Geometry check sheet. Reference: drawing and pictorial views, mm from the part's lowest x, y, z. Give positions to 0.01 mm unless a question says otherwise; leave off trailing zeros. Write each loop counter-clockwise with the first axis right and the second up, starting at its lowest first coordinate (ties: lowest second). Pieces come first, ordered by that corner, then holes. Notation, with made-up numbers: M -7.75,-12.75 L 29.25,-12.75 A13 ccw 29.25,-2.75 Z; hole C -38.5,74 d3. An arc over 180 degrees is marked long. One line per item, written item: value. Start each with the question number.
1. Cross-section at B-B on y = 1.75. Record the cut outline in (x, z), then the cut area to 3 significant figures.
2. Cross-section at D-D on x = 58. Record the cut outline in (y, z), then the cut area to 3 significant figures.
3. Cross-section at A-A on z = 11. Record the cut outline in (x, y), then the cut area to 3 significant figures.
4. Gauge pin test, flat end, axial feed: pin 1 (0.6 mm diameter, centred on x = 9.5, y = 4, fed in from +Z). Record the tip position at first contact, or that the pin passes through.
5. Scan lines: line 1 (X direction, y = 3, z = 16); line 2 (Z direction, x = 57, y = 3.5); line 3 (Y direction, x = 58, z = 37.75). Record each from-to range of solid material in increasing order.
6. Release check for a two-part mould opening along X. For the marked faces 1, 2 and 3 record: pulls with the +X half, pulls with the -X half, needs draft (parallel to the pull), parting line crosses it, or undercut.
7. Cross-section at C-C on z = 16.5. Record the cut outline in (x, y).
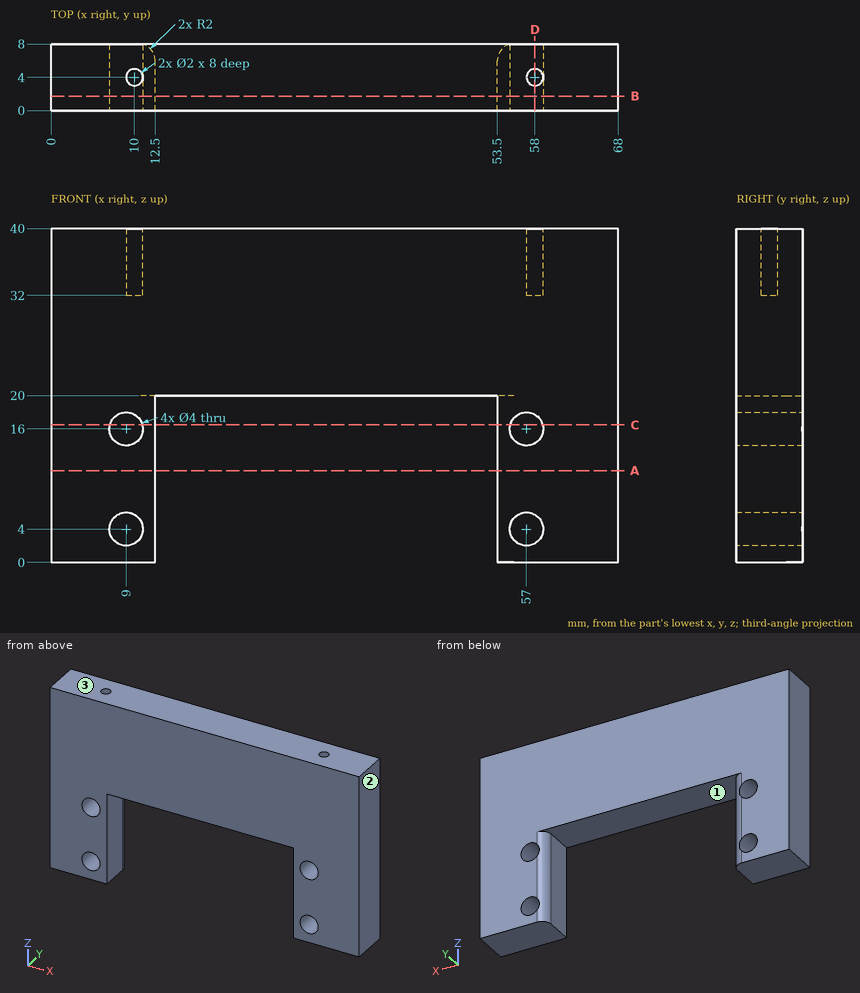
Report:
1. outline: M 0,0 L 12.5,0 L 12.5,20 L 53.5,20 L 53.5,0 L 68,0 L 68,40 L 0,40 Z; hole C 9,4 d4; hole C 9,16 d4; hole C 57,4 d4; hole C 57,16 d4
1. area: 1,850 mm^2
2. outline: M 0,0 L 8,0 L 8,2.27 L 0,2.27 Z; M 0,5.73 L 8,5.73 L 8,14.27 L 0,14.27 Z; M 0,17.73 L 8,17.73 L 8,40 L 5,40 L 5,32 L 3,32 L 3,40 L 0,40 Z
2. area: 249 mm^2
3. outline: M 0,0 L 12.5,0 L 12.5,6 A2 ccw 10.5,8 L 0,8 Z; M 53.5,0 L 68,0 L 68,8 L 55.5,8 A2 ccw 53.5,6 Z
3. area: 214 mm^2
4. pin 1: stops at z = 32
5. line 1: x = 0 to 7, 11 to 12.5, 53.5 to 55, 59 to 68
5. line 2: z = 0 to 2, 6 to 14, 18 to 40
5. line 3: y = 0 to 3, 5 to 8
6. face 1: undercut
6. face 2: pulls with the +X half
6. face 3: needs draft
7. outline: M 0,0 L 7.06,0 L 7.06,8 L 0,8 Z; M 10.94,0 L 12.5,0 L 12.5,6 A2 ccw 10.94,7.95 Z; M 53.5,0 L 55.06,0 L 55.06,7.95 A2 ccw 53.5,6 Z; M 58.94,0 L 68,0 L 68,8 L 58.94,8 Z
